For this review, take the finished solid that the model builds, in its own axes (mm). A direction names the side the tool comes from. Give positions to 0.01 mm unless a question says otherwise; leave off trailing zeros. Loops run counter-clockwise (first coordinate to the right, second up) from the corner with the lowest first, then second, coordinate; pieces in that order, holes last. Notation, with made-up numbers: (13.25, 28) - (70.25, 28) arc R12 cw to (70.25, 49) - close; hole circle Ø2 at (75, -31.75). An arc over 180 degrees is marked (long way). Answer in a Markdown table with one row per item.
```python
from build123d import *

# Parameters (mm, degrees)
SKETCH1_W           = 43.18
SKETCH1_H           = 35.56
BOSS_EXTRUDE1_DEPTH = 15.24
SKETCH2_W           = 33.02
SKETCH2_H           = 25.4
CUT_EXTRUDE1_DEPTH  = 9.525
SKETCH4_W           = 15.24
SKETCH4_H           = 15.24
CUT_EXTRUDE2_DEPTH  = 2.54
SKETCH7_R           = 1.27
CUT_EXTRUDE3_DEPTH  = 6.715
SKETCH8_R           = 1.27
CUT_EXTRUDE4_DEPTH  = 16.24


with BuildPart() as part:
    # Sketch1 → Boss-Extrude1 (new body)
    with BuildSketch(Plane(origin=(0, 0, 0), x_dir=(1, 0, 0), z_dir=(0, 1, 0))):
        with Locations((4.895164319, -9.074835681)):
            Rectangle(SKETCH1_W, SKETCH1_H)
    extrude(amount=BOSS_EXTRUDE1_DEPTH)

    # Sketch2 → Cut-Extrude1 (cut)
    with BuildSketch(Plane(origin=(0, 15.24, 0), x_dir=(1, 0, 0), z_dir=(0, 1, 0))):
        with Locations((4.895164319, -9.074835681)):
            Rectangle(SKETCH2_W, SKETCH2_H)
    extrude(amount=-CUT_EXTRUDE1_DEPTH, mode=Mode.SUBTRACT)

    # Sketch4 → Cut-Extrude2 (cut)
    with BuildSketch(Plane(origin=(0, 5.715, 0), x_dir=(1, 0, 0), z_dir=(0, 1, 0))):
        with Locations((4.895164319, -9.074835681)):
            Rectangle(SKETCH4_W, SKETCH4_H)
    extrude(amount=-CUT_EXTRUDE2_DEPTH, mode=Mode.SUBTRACT)

    # Sketch7 → Cut-Extrude3 (cut, through all)
    with BuildSketch(Plane(origin=(0, 5.715, 0), x_dir=(1, 0, 0), z_dir=(0, 1, 0))):
        with Locations((-5.264835681, -2.724835681)):
            Circle(SKETCH7_R)
        with Locations((-5.264835681, -15.424835681)):
            Circle(SKETCH7_R)
        with Locations((15.055164319, -2.724835681)):
            Circle(SKETCH7_R)
        with Locations((15.055164319, -15.424835681)):
            Circle(SKETCH7_R)
    extrude(amount=-CUT_EXTRUDE3_DEPTH, mode=Mode.SUBTRACT)

    # Sketch8 → Cut-Extrude4 (cut, through all)
    with BuildSketch(Plane(origin=(0, 15.24, 0), x_dir=(1, 0, 0), z_dir=(0, 1, 0))):
        with Locations((-14.154835681, 6.165164319)):
            Circle(SKETCH8_R)
        with Locations((-14.154835681, -24.353191234)):
            Circle(SKETCH8_R)
        with Locations((23.945164319, 6.165164319)):
            Circle(SKETCH8_R)
        with Locations((23.945164319, -24.314835681)):
            Circle(SKETCH8_R)
    extrude(amount=-CUT_EXTRUDE4_DEPTH, mode=Mode.SUBTRACT)


solid = part.part
```
1. Mouldability with a two-part tool opening along X and no side actions: class faces 3 (the face through (5, 4, 1.455)), 4 (the face through (26.485, 8, 9)), 5 (the face through (5, 8, -8.705)), 6 (the face through (-13.57, 7.73, 25.48)) as released by +X, released by -X, zero draft, split by the parting line, or undercut.
Values:
| item | result |
|---|---|
| face 3 | undercut |
| face 4 | released by +X |
| face 5 | zero draft |
| face 6 | undercut |
2. We need section C-C, the plane y = 1.5. Count the separate pieces of the cut face and the enclosed holes in it, and give its area (3 significant figures).
Values:
| item | result |
|---|---|
| separate pieces | 1 |
| enclosed holes | 8 |
| area | 1,490 mm^2 |
3. For faces 1 (the face through (-16.695, 8, 9)), 2 (the face through (5, 11, 21.775)), list the 3-axis set-ups (+Z, -Z, +X, -X, +Y, -Y) from which the entire face can be reached by the end or side of a thin tool; tool diameter is ignored.
Values:
| item | result |
|---|---|
| face 1 | +Z, -Z, -X, +Y, -Y |
| face 2 | +Y |
4. Clearance check with flat-ended pins moving along their axes: pin 1 (3.5 mm diameter, centred on x = -5.26, z = 2.72, fed in from +Y) (3 decimals); pin 2 (1.5 mm diameter, centred on x = 23.95, z = -6.17, fed in from -Y). State where each tip first meets the part, or that it passes through.
Values:
| item | result |
|---|---|
| pin 1 | stops at y = 5.715 |
| pin 2 | passes through |
5. Wall thickness on line 1 (Z direction, x = 12.5, y = 8.25); line 2 (X direction, y = 2.5, z = 24.5); line 3 (X direction, y = 14.75, z = 13.5): over which ranges is each line inside the solid? List them lowest first. Write a range as [from, to].
Values:
| item | result |
|---|---|
| line 1 | z = [-8.71, -3.63], [21.77, 26.85] |
| line 2 | x = [-16.69, -15.42], [-12.89, 22.69], [25.2, 26.49] |
| line 3 | x = [-16.69, -11.61], [21.41, 26.49] |
6. We need section A-A, the plane z = 20.5. Give the boundary of the cut face in (x, y) (3 decimals), and give its area (3 significant figures).
Values:
| item | result |
|---|---|
| outline | (-16.695, 0) - (26.485, 0) - (26.485, 15.24) - (21.405, 15.24) - (21.405, 5.715) - (-11.615, 5.715) - (-11.615, 15.24) - (-16.695, 15.24) - close |
| area | 344 mm^2 |
7. We need section B-B, the plane x = 1.5. Give the boundary of the cut face in (y, z) (3 decimals), and give its area (3 significant figures).
Values:
| item | result |
|---|---|
| outline | (0, -8.705) - (15.24, -8.705) - (15.24, -3.625) - (5.715, -3.625) - (5.715, 1.455) - (3.175, 1.455) - (3.175, 16.695) - (5.715, 16.695) - (5.715, 21.775) - (15.24, 21.775) - (15.24, 26.855) - (0, 26.855) - close |
| area | 261 mm^2 |
